Part model, mm, in its own coordinate system. Round coordinates to 2 decimals unless told otherwise and drop trailing zeros. Write each loop counter-clockwise with the first axis right and the second up, starting at its lowest first coordinate (ties: lowest second). Pieces come first, ordered by that corner, then holes.
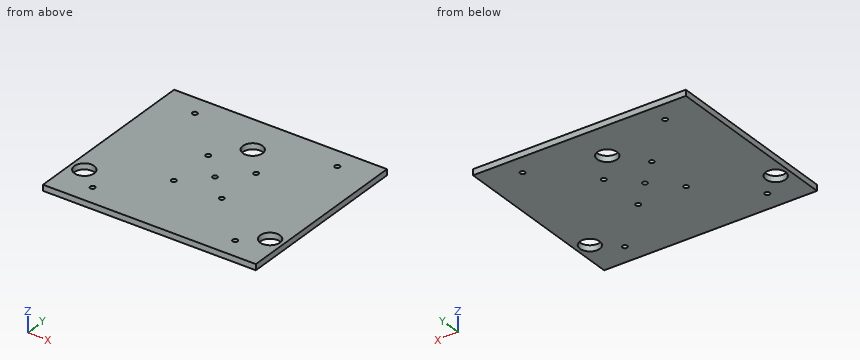
Autodesk Fusion 360 part; units mm, degrees
sketch "movingPlatform" plane through (0, 0, 0) normal (0, 0, 1) x (1, 0, 0)
  line L0 (-68.75, 59) -> (68.75, 59)
  line L1 (68.75, 59) -> (68.75, -59)
  line L2 (68.75, -59) -> (-68.75, -59)
  line L3 (-68.75, -59) -> (-68.75, 59)
  line L4 (-68.75, 59) -> (68.75, -59) construction
  line L5 (68.75, 59) -> (-68.75, -59) construction
  circle A0 centre (-60, -34) radius 6.4
  line L6 (0, 2.5) -> (0, 20)
  circle A1 centre (60, -34) radius 6.4
  circle A2 centre (0, 34) radius 6.4
  circle A3 centre (-46, -46) radius 1.588
  circle A4 centre (-15.5, -15.5) radius 1.588
  circle A5 centre (0, 0) radius 57 construction
  circle A6 centre (15.5, -15.5) radius 1.588
  circle A7 centre (15.5, 15.5) radius 1.588
  circle A8 centre (46, -46) radius 1.588
  circle A9 centre (-46, 46) radius 1.588
  circle A10 centre (46, 46) radius 1.588
  circle A11 centre (-15.5, 15.5) radius 1.588
  circle A12 centre (0, 0) radius 1.588
  dimension "d1" = 137.5
  dimension "d2" = 118
  dimension "d3" = 12.8
  dimension "d4" = 120
  dimension "d5" = 12.8
  dimension "d6" = 68
  dimension "d7" = 25
  dimension "d8" = 25
  dimension "d9" = 3.176
  dimension "d12" = 92
  dimension "d13" = 92
  dimension "d21" = 3.176
  dimension "d24" = 31
  dimension "d25" = 31
  dimension "d27" = 15.5
  dimension "d31" = 114
  dimension "d34" = 46
  dimension "d37" = 46
  dimension "d49" = 15.5
  dimension "d52" = 3.176
extrude "Extrude3" add sketch "movingPlatform" along normal blind 3.8
equation "d4 = 132.800 mm - 12.8 mm"
Q1. Saw through at C-C, the plane x = 0. Write the cut outline in (y, z).
Q2. Saw through at A-A, the plane y = 34. Write the cut outline in (x, z).
Q3. Saw through at D-D, the plane z = 1.2. Give the number of separate pieces and of enclosed holes in the cut face, and give its area (3 significant figures).
Q4. Saw through at B-B, the plane y = -34. Write the cut outline in (x, z).
Q5. Wall check: line 1 (Y direction, x = -46, z = 1.5); line 2 (Y direction, x = 60, z = 1.1); line 3 (X direction, y = -39.5, z = 0.6). Give the ranges that are in metal, low to high.
Computed:
1. outline: (-59, 0) - (-1.59, 0) - (-1.59, 3.8) - (-59, 3.8) - close; (1.59, 0) - (27.6, 0) - (27.6, 3.8) - (1.59, 3.8) - close; (40.4, 0) - (59, 0) - (59, 3.8) - (40.4, 3.8) - close
2. outline: (-68.75, 0) - (-6.4, 0) - (-6.4, 3.8) - (-68.75, 3.8) - close; (6.4, 0) - (68.75, 0) - (68.75, 3.8) - (6.4, 3.8) - close
3. separate pieces: 1
3. enclosed holes: 12
3. area: 15,800 mm2
4. outline: (-68.75, 0) - (-66.4, 0) - (-66.4, 3.8) - (-68.75, 3.8) - close; (-53.6, 0) - (53.6, 0) - (53.6, 3.8) - (-53.6, 3.8) - close; (66.4, 0) - (68.75, 0) - (68.75, 3.8) - (66.4, 3.8) - close
5. line 1: y = -59 to -47.59, -44.41 to 44.41, 47.59 to 59
5. line 2: y = -59 to -40.4, -27.6 to 59
5. line 3: x = -68.75 to -63.27, -56.73 to 56.73, 63.27 to 68.75
